from build123d import *

# Parameters (mm, degrees)
SKETCH1_W            = 48.254
SKETCH1_H            = 3
BOSS_EXTRUDE1_DEPTH  = 70
BOSS_EXTRUDE3_DEPTH  = 8
BOSS_EXTRUDE4_DEPTH  = 8
BOSS_EXTRUDE5_DEPTH  = 8
BOSS_EXTRUDE6_DEPTH  = 70
SKETCH7_W            = 40.394634483
SKETCH7_H            = 17
CUT_EXTRUDE3_DEPTH   = 70
BOSS_EXTRUDE7_DEPTH  = 70
BOSS_EXTRUDE10_DEPTH = 8
BOSS_EXTRUDE11_DEPTH = 70
SKETCH13_W           = 83.001411072
SKETCH13_H           = 87.868559997
CUT_EXTRUDE4_DEPTH   = 4
SKETCH14_W           = 48.254
SKETCH14_H           = 10
BOSS_EXTRUDE12_DEPTH = 20
SKETCH16_W           = 56.254
SKETCH16_H           = 5
CUT_EXTRUDE5_DEPTH   = 100
SKETCH17_W           = 15
SKETCH17_H           = 15
BOSS_EXTRUDE14_DEPTH = 13
CUT_EXTRUDE8_DEPTH   = 5
SKETCH21_R           = 2.3
CUT_EXTRUDE9_DEPTH   = 15
SKETCH23_W           = 12
SKETCH23_H           = 40.530858039
CUT_EXTRUDE10_DEPTH  = 9
SKETCH25_R           = 2.3
CUT_EXTRUDE11_DEPTH  = 20
SKETCH26_R           = 2.3
CUT_EXTRUDE12_DEPTH  = 20
BOSS_EXTRUDE16_DEPTH = 20
SKETCH28_W           = 15
SKETCH28_H           = 15
BOSS_EXTRUDE17_DEPTH = 10
SKETCH29_R           = 2.3
CUT_EXTRUDE13_DEPTH  = 20
SKETCH30_W           = 10.391026801
SKETCH30_H           = 12
BOSS_EXTRUDE18_DEPTH = 5
SKETCH31_R           = 2.3
CUT_EXTRUDE14_DEPTH  = 45
SKETCH36_R           = 60.036471347
CUT_EXTRUDE15_DEPTH  = 2
SKETCH37_W           = 5
SKETCH37_H           = 88
BOSS_EXTRUDE19_DEPTH = 10
CUT_EXTRUDE16_DEPTH  = 5
SKETCH39_R           = 2.1
CUT_EXTRUDE17_DEPTH  = 5
SKETCH40_W           = 55
SKETCH40_H           = 46.30826584
CUT_EXTRUDE18_DEPTH  = 5


with BuildPart() as part:
    # Sketch1 → Boss-Extrude1 (new body)
    with BuildSketch(Plane.XY):
        Polygon((4, 0), (0, 0), (0, 70), (56.254, 70), (56.254, 0), (52.254, 0), (52.254, 65), (4, 65), align=None)
        with Locations((28.127, 53.5)):
            Rectangle(SKETCH1_W, SKETCH1_H)
    extrude(amount=BOSS_EXTRUDE1_DEPTH)

    # Sketch3 → Boss-Extrude3 (add)
    with BuildSketch(Plane.XY.offset(70)):
        Polygon((0, 62.5), (0, 70), (-40.394634483, 70), (0, 0.034440722), (0, 17.466679003), (-26, 62.5), align=None)
    extrude(amount=-BOSS_EXTRUDE3_DEPTH)

    # Sketch4 → Boss-Extrude4 (add)
    with BuildSketch(Plane(origin=(0, 0, 0), x_dir=(-1, 0, 0), z_dir=(0, 0, -1))):
        Polygon((0, 70), (40.394634483, 70), (0, 0), (0, 17.466679003), (26, 62.5), (0, 62.5), align=None)
    extrude(amount=-BOSS_EXTRUDE4_DEPTH)

    # Sketch5 → Boss-Extrude5 (add)
    with BuildSketch(Plane(origin=(0, 0, 39), x_dir=(-1, 0, 0), z_dir=(0, 0, -1))):
        Polygon((0, 62.5), (0, 70), (40.394634483, 70), (0, 0), (0, 17.466679003), (26, 62.5), align=None)
    extrude(amount=BOSS_EXTRUDE5_DEPTH)

    # Sketch6 → Boss-Extrude6 (add)
    with BuildSketch(Plane(origin=(0, 0, 0), x_dir=(-1, 0, 0), z_dir=(0, 0, -1))):
        Polygon((0, 62.5), (36.066637932, 62.5), (40.394634483, 70), (0, 70), align=None)
        Polygon((-4, 0), (0, 0), (7.50186069, 13), (-4, 13), align=None)
    extrude(amount=-BOSS_EXTRUDE6_DEPTH)

    # Sketch7 → Cut-Extrude3 (cut)
    with BuildSketch(Plane.XY.offset(70)):
        with Locations((-20.197317242, 61.5)):
            Rectangle(SKETCH7_W, SKETCH7_H)
    extrude(amount=-CUT_EXTRUDE3_DEPTH, mode=Mode.SUBTRACT)

    # Sketch8 → Boss-Extrude7 (add)
    with BuildSketch(Plane(origin=(0, 0, 0), x_dir=(-1, 0, 0), z_dir=(0, 0, -1))):
        Polygon((-4, 55), (-4, 52), (30.007442759, 52), (31.73864138, 55), align=None)
    extrude(amount=-BOSS_EXTRUDE7_DEPTH)

    # Sketch11 → Boss-Extrude10 (add)
    with BuildSketch(Plane.XY.offset(70)):
        Polygon((-31.73864138, 55), (0, 0), (-3.053687451, 13), (-27.288965695, 55), align=None)
    extrude(amount=-BOSS_EXTRUDE10_DEPTH)

    # Sketch12 → Boss-Extrude11 (add)
    with BuildSketch(Plane.XY.offset(70)):
        Polygon((-31.73864138, 55), (-27.75981023, 48.105069917), (0, 48.105069917), (0, 55), align=None)
    extrude(amount=-BOSS_EXTRUDE11_DEPTH)

    # Sketch13 → Cut-Extrude4 (cut)
    with BuildSketch(Plane.XZ):
        with Locations((25.938658228, 33.313825886)):
            Rectangle(SKETCH13_W, SKETCH13_H)
    extrude(amount=-CUT_EXTRUDE4_DEPTH, mode=Mode.SUBTRACT)

    # Sketch14 → Boss-Extrude12 (add)
    with BuildSketch(Plane.XY.offset(70)):
        Polygon((-2.308264828, 4), (-31.73864138, 55), (0, 55), (0, 70), (56.254, 70), (56.254, 4), (52.254, 4), (52.254, 52), (4, 52), (4, 4), align=None)
        Polygon((-17.689083241, 48.105069917), (0, 48.105069917), (0, 17.466679003), align=None, mode=Mode.SUBTRACT)
        with Locations((28.127, 60)):
            Rectangle(SKETCH14_W, SKETCH14_H, mode=Mode.SUBTRACT)
    extrude(amount=BOSS_EXTRUDE12_DEPTH)

    # Sketch16 → Cut-Extrude5 (cut)
    with BuildSketch(Plane.XY.offset(90)):
        with Locations((28.127, 67.5)):
            Rectangle(SKETCH16_W, SKETCH16_H)
    extrude(amount=-CUT_EXTRUDE5_DEPTH, mode=Mode.SUBTRACT)

    # Sketch17 → Boss-Extrude14 (add)
    with BuildSketch(Plane(origin=(0, 65, 0), x_dir=(1, 0, 0), z_dir=(0, 1, 0))):
        with Locations((44.754, -7.5)):
            Rectangle(SKETCH17_W, SKETCH17_H)
        with Locations((44.754, -82.5)):
            Rectangle(SKETCH17_W, SKETCH17_H)
    extrude(amount=-BOSS_EXTRUDE14_DEPTH)

    # Sketch22 → Cut-Extrude8 (cut)
    with BuildSketch(Plane.XZ.offset(-52)):
        Polygon((48.096455918, 6.003620146), (47.904143628, 10.329474511), (44.06168771, 12.325854365), (40.411544082, 9.996379854), (40.603856372, 5.670525489), (44.44631229, 3.674145635), align=None)
        Polygon((45.200685086, 75.774625774), (48.386623963, 78.707166221), (47.439938877, 82.932540447), (43.307314914, 84.225374226), (40.121376037, 81.292833779), (41.068061123, 77.067459553), align=None)
    extrude(amount=-CUT_EXTRUDE8_DEPTH, mode=Mode.SUBTRACT)

    # Sketch21 → Cut-Extrude9 (cut)
    with BuildSketch(Plane(origin=(0, 52, 0), x_dir=(-1, 0, 0), z_dir=(0, -1, 0))):
        with Locations(Location((-44.254, -80, 0), (0, 0, 90))):
            Circle(SKETCH21_R)
        with Locations(Location((-44.254, -8, 0), (0, 0, 90))):
            Circle(SKETCH21_R)
    extrude(amount=-CUT_EXTRUDE9_DEPTH, mode=Mode.SUBTRACT)

    # Sketch23 → Cut-Extrude10 (cut)
    with BuildSketch(Plane(origin=(0, 0, 0), x_dir=(0, 0, 1), z_dir=(-0.8661319205837115, -0.49981546209173167, 0))):
        with Locations((76, 35.274689955)):
            Rectangle(SKETCH23_W, SKETCH23_H)
    extrude(amount=-CUT_EXTRUDE10_DEPTH, mode=Mode.SUBTRACT)

    # Sketch25 → Cut-Extrude11 (cut)
    with BuildSketch(Plane(origin=(0, 48.105069917, 0), x_dir=(-1, 0, 0), z_dir=(0, -1, 0))):
        with Locations(Location((17.075514089, -19.30064897, 0), (0, 0, 90))):
            Circle(SKETCH25_R)
        with Locations(Location((17.075514089, -50.613733273, 0), (0, 0, 90))):
            Circle(SKETCH25_R)
    extrude(amount=-CUT_EXTRUDE11_DEPTH, mode=Mode.SUBTRACT)

    # Sketch26 → Cut-Extrude12 (cut)
    with BuildSketch(Plane.XZ.offset(-48.105069917)):
        with Locations(Location((-17.075514089, 75.391336138, 0), (0, 0, 262.674363606))):
            Circle(SKETCH26_R)
    extrude(amount=-CUT_EXTRUDE12_DEPTH, mode=Mode.SUBTRACT)

    # Sketch27 → Boss-Extrude16 (add)
    with BuildSketch(Plane.XY.offset(90)):
        Polygon((-23.310381194, 48.105069917), (-27.75981023, 48.105069917), (-31.73864138, 55), (-23.310381194, 55), align=None)
    extrude(amount=-BOSS_EXTRUDE16_DEPTH)

    # Sketch28 → Boss-Extrude17 (add)
    with BuildSketch(Plane(origin=(0, 55, 0), x_dir=(1, 0, 0), z_dir=(0, 1, 0))):
        with Locations((11.5, -7.5)):
            Rectangle(SKETCH28_W, SKETCH28_H)
        with Locations((11.5, -82.5)):
            Rectangle(SKETCH28_W, SKETCH28_H)
    extrude(amount=BOSS_EXTRUDE17_DEPTH)

    # Sketch29 → Cut-Extrude13 (cut)
    with BuildSketch(Plane(origin=(0, 52, 0), x_dir=(-1, 0, 0), z_dir=(0, -1, 0))):
        with Locations(Location((-12.254, -8, 0), (0, 0, 90))):
            Circle(SKETCH29_R)
        with Locations(Location((-12.254, -80, 0), (0, 0, 90))):
            Circle(SKETCH29_R)
    extrude(amount=-CUT_EXTRUDE13_DEPTH, mode=Mode.SUBTRACT)

    # Sketch30 → Boss-Extrude18 (add)
    with BuildSketch(Plane.XZ.offset(-48.105069917)):
        with Locations((-22.56429683, 76)):
            Rectangle(SKETCH30_W, SKETCH30_H)
    extrude(amount=-BOSS_EXTRUDE18_DEPTH)

    # Sketch31 → Cut-Extrude14 (cut)
    with BuildSketch(Plane.XZ.offset(-48.105069917)):
        with Locations(Location((-17.075514089, 75.391336138, 0), (0, 0, 270))):
            Circle(SKETCH31_R)
    extrude(amount=-CUT_EXTRUDE14_DEPTH, mode=Mode.SUBTRACT)

    # Sketch36 → Cut-Extrude15 (cut)
    with BuildSketch(Plane.XY.offset(90)):
        with Locations((23.036116276, 36.93280147)):
            Circle(SKETCH36_R)
    extrude(amount=-CUT_EXTRUDE15_DEPTH, mode=Mode.SUBTRACT)

    # Sketch37 → Boss-Extrude19 (add)
    with BuildSketch(Plane(origin=(0, 55, 0), x_dir=(1, 0, 0), z_dir=(0, 1, 0))):
        with Locations((-29.23864138, -44)):
            Rectangle(SKETCH37_W, SKETCH37_H)
    extrude(amount=BOSS_EXTRUDE19_DEPTH)

    # Sketch38 → Cut-Extrude16 (cut)
    with BuildSketch(Plane.XZ.offset(-52)):
        Polygon((12.254, 75.669872981), (16.004, 77.834936491), (16.004, 82.165063509), (12.254, 84.330127019), (8.504, 82.165063509), (8.504, 77.834936491), align=None)
        Polygon((15.567298341, 5.212159598), (16.32498978, 9.475480332), (13.011691439, 12.263320734), (8.940701659, 10.787840402), (8.18301022, 6.524519668), (11.496308561, 3.736679266), align=None)
    extrude(amount=-CUT_EXTRUDE16_DEPTH, mode=Mode.SUBTRACT)

    # Sketch39 → Cut-Extrude17 (cut)
    with BuildSketch(Plane(origin=(4, 0, 0), x_dir=(0, 0, -1), z_dir=(1, 0, 0))):
        with Locations(Location((-47.514718626, 36.485281374, 0), (0, 0, 90))):
            Circle(SKETCH39_R)
        with Locations(Location((-48, 20, 0), (0, 0, 90))):
            Circle(SKETCH39_R)
        with Locations(Location((-16.485281374, 19.514718626, 0), (0, 0, 90))):
            Circle(SKETCH39_R)
        with Locations(Location((-16.485281374, 36.485281374, 0), (0, 0, 90))):
            Circle(SKETCH39_R)
    extrude(amount=-CUT_EXTRUDE17_DEPTH, mode=Mode.SUBTRACT)

    # Sketch40 → Cut-Extrude18 (cut)
    with BuildSketch(Plane(origin=(56.254, 0, 0), x_dir=(0, 0, -1), z_dir=(1, 0, 0))):
        with Locations((-60.5, 27.15413292)):
            Rectangle(SKETCH40_W, SKETCH40_H)
    extrude(amount=-CUT_EXTRUDE18_DEPTH, mode=Mode.SUBTRACT)


solid = part.part
Verification items for the finished model (mm, model axes). A direction names the side the tool comes from. Coordinates: 2 decimals unless noted, no trailing zeros. Order: outer loops, then holes, each group sorted by start corner. A loop starts at its lowest first (then second) coordinate and runs counter-clockwise, first axis right, second up. Notation, with made-up numbers: M 74,-17.5 L 133,-17.5 A27 cw 133,6.5 Z; hole C 63,-14 d7. An arc over 180 degrees is marked long. One line per item, written item: value. Start each with the question number.
Item 1: Sectioned sample at B-B on y = 32. Record the cut outline in (x, z).
Item 2: Sectioned sample at C-C on y = 9.5. Record the cut outline in (x, z).
Item 3: Thickness scan on probe 1 along X at (y, z) = (56, 84.5); probe 2 along X at (y, z) = (62.5, 54); probe 3 along Y at (x, z) = (-1.5, 57.5). Record the ranges inside material, lowest first.
Item 4: Depth check by flat-ended pin: P1, Ø6.5, axis at x = 45, z = 80.5, coming from the -Y side; P2, Ø1.2, axis at x = 54.5, z = 55, coming from the -Y side; P3, Ø3, axis at y = 43.5, z = 54.5, coming from the +X side. Enter the tip coordinate at first touch or a pass-through.
Item 5: Sectioned sample at D-D on x = -25. Record the cut outline in (y, z), then the cut area to 3 significant figures.
Item 6: Access from +Z, -Z, +X, -X, +Y, -Y to the whole of each face (thin tool, end or side, straight path). Record for faces 1 (the cylindrical face through (42.214, 60.944, 78.939)), 2 (the flat face through (52.254, 60, 45)), 3 (the flat face through (37.254, 60, 8)), 4 (the flat face through (10.5, 57, 78.1)), 5 (the flat face through (-8.72, 32.57, 66.06)).
Item 7: Mould release check, pull along Y, two halves, no side actions. Record for faces 6 (the flat face through (45, 60, 75)), 7 (the flat face through (28, 52, 43)), 8 (the flat face through (-14, 33, 82)), 9 (the flat face through (-3.659, 15.218, 75.916)): pulls with the +Y half, pulls with the -Y half, needs draft (parallel to the pull), parting line crosses it, or undercut.
Item 8: Sectioned sample at A-A on z = 64. Record the cut outline in (x, y), then the cut area to 3 significant figures.
Calculated:
1. outline: M -18.47,0 L -8.39,0 L -8.39,8 L -18.47,8 Z; M -18.47,31 L -8.39,31 L -8.39,39 L -18.47,39 Z; M -18.47,62 L -8.39,62 L -8.39,70 L -18.47,70 Z; M -18.47,82 L -8.39,82 L -8.39,88 L -18.47,88 Z; M 0,0 L 4,0 L 4,88 L 0,88 Z; M 52.25,0 L 56.25,0 L 56.25,33 L 52.25,33 Z
2. outline: M -5.48,0 L 4,0 L 4,88 L -5.48,88 Z; M 52.25,0 L 56.25,0 L 56.25,33 L 52.25,33 Z
3. probe 1: -31.74 to -26.74, 0 to 19, 37.25 to 56.25
3. probe 2: -31.74 to -26.74, 0 to 4, 52.25 to 56.25
3. probe 3: 4 to 13, 48.11 to 55
4. P1: y = 52
4. P2: y = 50.31
4. P3: x = 4
5. outline: M 43.32,0 L 55,0 L 55,88 L 43.32,88 L 43.32,82 L 48.11,82 L 48.11,70 L 43.32,70 L 43.32,62 L 48.11,62 L 48.11,39 L 43.32,39 L 43.32,31 L 48.11,31 L 48.11,8 L 43.32,8 Z
5. area: 750 mm^2
6. face 1: +Y, -Y
6. face 2: +Y
6. face 3: +Z, -Z, +Y
6. face 4: -Y
6. face 5: +Z, -Z
7. face 6: needs draft
7. face 7: pulls with the -Y half
7. face 8: undercut
7. face 9: undercut
8. outline: M -31.74,55 L -2.31,4 L 4,4 L 4,52 L 52.25,52 L 52.25,50.31 L 56.25,50.31 L 56.25,65 L 52.25,65 L 52.25,55 L 4,55 L 4,65 L 0,65 L 0,55 L -26.74,55 L -26.74,65 L -31.74,65 Z; hole M -17.69,48.11 L 0,17.47 L 0,48.11 Z
8. area: 1,090 mm^2
